The listing builds one solid part. Answer for the finished solid, in the listing's coordinates (mm). A direction names the side the tool comes from. Give positions to 0.01 mm unless a question says otherwise; leave off trailing zeros. Loops run counter-clockwise (first coordinate to the right, second up) from the corner with the lowest first, then second, coordinate; pieces in that order, holes last. Notation, with made-up numbers: (-31.5, 29.25) - (-3.5, 29.25) arc R12 ccw to (-3.5, 34.25) - close; hole circle Ø2 at (65.5, 87.25). An arc over 180 degrees is marked (long way). Write item = value, one per line. Start each with the question number.
1) The part is cut by section A-A on z = -6. Write down the section's boundary in (x, y).
2) The part is cut by section C-C on y = -8.75. Write down the section's boundary in (x, z).
3) The part is cut by section B-B on x = -1.5. Write down the section's boundary in (y, z).
4) Which of the six approach directions +Z, -Z, +X, -X, +Y, -Y give full straight-line access (tool end or side, diameter ignored) to faces 1 (the flat face through (-2, 0, 0)), 2 (the flat face through (0, -14, 17.5)), 3 (the flat face through (2, 0, 0))?
5) Consider probe 1 along X at (y, z) = (-26.5, -5); probe 2 along Y at (x, z) = (-2, -12); probe 3 along Y at (x, z) = (-0.5, 14). Determine where each line is inside the solid, lowest interval first.
6) Flat-ended cylindrical pins translate along their axes: P1, Ø5, axis at y = -18.5, z = -9, coming from the -X side; P2, Ø1.4, axis at x = 2, z = -3.5, coming from the -Y side; P3, Ø3, axis at y = -3.5, z = 1, coming from the +X side. Find the tip coordinate at first contact, or state that the pin passes through.
from build123d import *

# Parameters (mm, degrees)
F0_W     = 2.25
F0_H     = 35
F0_W_2   = 1.5
F1_DEPTH = 1
F2_DEPTH = 28
F3_R     = 0.5
F4_R     = 0.75


with BuildPart() as f1:
    # F0 (on Front) → F1 (new body)
    with BuildSketch(Plane.XZ):
        with Locations((1.875, 0)):
            Rectangle(F0_W, F0_H)
        Rectangle(F0_W_2, F0_H)
        with Locations((-1.875, 0)):
            Rectangle(F0_W, F0_H)
    extrude(amount=-F1_DEPTH)

    # F0 (on Front) → F2 (join)
    with BuildSketch(Plane.XZ):
        Rectangle(F0_W_2, F0_H)
    extrude(amount=F2_DEPTH)

    # F3
    f3_edges = [f1.edges().sort_by_distance(p)[0] for p in [
        (-3, 0, 0),
        (3, 0, 0),
        (-0.75, -28, 0),
        (0.75, -28, 0),
    ]]
    fillet(f3_edges, radius=F3_R)

    # F4
    f4_edges = [f1.edges().sort_by_distance(p)[0] for p in [
        (0, 1, 17.5),
        (0, 1, -17.5),
    ]]
    fillet(f4_edges, radius=F4_R)


solid = f1.part
Answer below:
q1.outline = (-3, 0.5) arc R0.5 ccw to (-2.5, 0) - (-0.75, 0) - (-0.75, -27.5) arc R0.5 ccw to (-0.25, -28) - (0.25, -28) arc R0.5 ccw to (0.75, -27.5) - (0.75, 0) - (2.5, 0) arc R0.5 ccw to (3, 0.5) - (3, 1) - (-3, 1) - close
q2.outline = (-0.75, -17.5) - (0.75, -17.5) - (0.75, 17.5) - (-0.75, 17.5) - close
q3.outline = (0, -17.5) - (0.25, -17.5) arc R0.75 ccw to (1, -16.75) - (1, 16.75) arc R0.75 ccw to (0.25, 17.5) - (0, 17.5) - close
q4.face_1 = +Z, -Z, -X, -Y
q4.face_2 = +Z, +X, -X, +Y, -Y
q4.face_3 = +Z, -Z, +X, -Y
q5.probe_1 = -0.75 to 0.75
q5.probe_2 = 0 to 1
q5.probe_3 = -27.93 to 1
q6.P1 = -0.75
q6.P2 = 0
q6.P3 = 0.75
